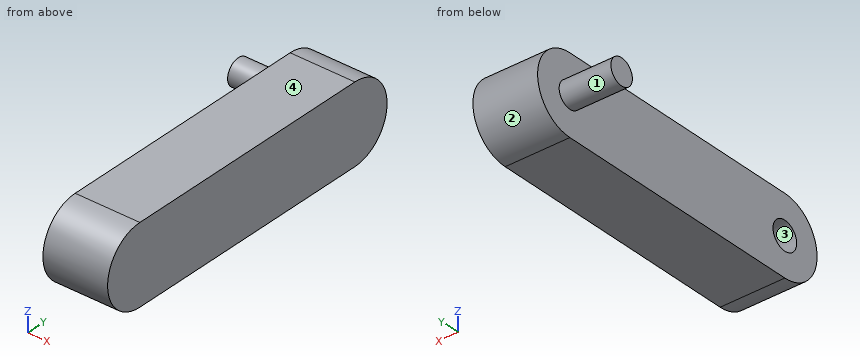
from build123d import *

# Parameters (mm, degrees)
BOSS_EXTRUDE1_DEPTH = 63.5
SKETCH2_R           = 13.97
CUT_EXTRUDE1_DEPTH  = 48.26
SKETCH3_R           = 12.7
BOSS_EXTRUDE2_DEPTH = 50.8


with BuildPart() as part:
    # Sketch1 → Boss-Extrude1 (new body)
    with BuildSketch(Plane(origin=(0, 0, 0), x_dir=(0, 0, -1), z_dir=(1, 0, 0))):
        with BuildLine():
            Line((38.1, 127), (38.1, -127))
            ThreePointArc((38.1, -127), (0, -165.1), (-38.1, -127))
            Line((-38.1, -127), (-38.1, 127))
            ThreePointArc((-38.1, 127), (0, 165.1), (38.1, 127))
        make_face()
    extrude(amount=BOSS_EXTRUDE1_DEPTH)

    # Sketch2 → Cut-Extrude1 (cut)
    with BuildSketch(Plane(origin=(0, 0, 0), x_dir=(0, 0, -1), z_dir=(1, 0, 0))):
        with Locations(Location((0, -127, 0), (0, 0, 180))):
            Circle(SKETCH2_R)
    extrude(amount=CUT_EXTRUDE1_DEPTH, mode=Mode.SUBTRACT)

    # Sketch3 → Boss-Extrude2 (add)
    with BuildSketch(Plane(origin=(0, 0, 0), x_dir=(0, 0, -1), z_dir=(1, 0, 0))):
        with Locations((0, 127)):
            Circle(SKETCH3_R)
    extrude(amount=-BOSS_EXTRUDE2_DEPTH)


solid = part.part
Read the model definition and answer for the solid it produces. Units are mm, in the model's axes. Face numbers are marked on the shaded views. Round coordinates to 2 decimals unless told otherwise and drop trailing zeros. Write each loop counter-clockwise with the first axis right and the second up, starting at its lowest first coordinate (ties: lowest second). Pieces come first, ordered by that corner, then holes. Notation, with made-up numbers: (-27, 40) - (15, 40) arc R20 cw to (15, 77) - close; hole circle Ø10 at (35, 8.25). An arc over 180 degrees is marked (long way). Use a Markdown table: item, result.
(1) The part is cut by section A-A (z = 0). Write down the section's boundary in (x, y).
Reported:
| item | result |
|---|---|
| outline | (-50.8, 114.3) - (0, 114.3) - (0, -113.03) - (48.26, -113.03) - (48.26, -140.97) - (0, -140.97) - (0, -165.1) - (63.5, -165.1) - (63.5, 165.1) - (0, 165.1) - (0, 139.7) - (-50.8, 139.7) - close |
(2) The part is cut by section B-B (x = 32). Write down the section's boundary in (y, z), then the cut area to 3 significant figures.
Reported:
| item | result |
|---|---|
| outline | (-127, -38.1) - (127, -38.1) arc R38.1 ccw to (127, 38.1) - (-127, 38.1) arc R38.1 ccw to start; hole circle Ø27.94 at (-127, 0) |
| area | 23,300 mm2 |
(3) Straight lines are drawn through the part: line 1 along Y through (x, z) = (32, 0); line 2 along Z through (x, y) = (32.5, -127); line 3 along X through (y, z) = (-15, 3.5). For each, find the intervals that lie inside material, in ascending order. Write a range as [from, to].
Reported:
| item | result |
|---|---|
| line 1 | [-165.1, -140.97], [-113.03, 165.1] |
| line 2 | [-38.1, -13.97], [13.97, 38.1] |
| line 3 | [0, 63.5] |
(4) Each of these flat-tipped pins is pushed along its axis until it touches: pin 1 Ø12 at (x, z) = (-26, 12.5) entering from -Y; pin 2 Ø23 at (y, z) = (36.5, 3.5) entering from -X; pin 3 Ø1.5 at (x, z) = (-32.5, -1) entering from -Y. Where does it stop, or does it pass through?
Reported:
| item | result |
|---|---|
| pin 1 | y = 116.09 |
| pin 2 | x = 0 |
| pin 3 | y = 114.3 |
(5) The part is cut by section C-C (y = 26). Write down the section's boundary in (x, z), then the cut area to 3 significant figures.
Reported:
| item | result |
|---|---|
| outline | (0, -38.1) - (63.5, -38.1) - (63.5, 38.1) - (0, 38.1) - close |
| area | 4,840 mm2 |
(6) The mould has two halves that part along Y. Classify the marked faces 1, 2, 3 and 4: released by +Y, released by -Y, zero draft, split by the parting line, or undercut.
Reported:
| item | result |
|---|---|
| face 1 | split by the parting line |
| face 2 | released by +Y |
| face 3 | undercut |
| face 4 | zero draft |
(7) The part is cut by section D-D (x = -15.5). Write down the section's boundary in (y, z), then the cut area to 3 significant figures.
Reported:
| item | result |
|---|---|
| outline | circle Ø25.4 at (127, 0) |
| area | 507 mm2 |
